Can you work these out from the model? Positions are in its coordinate system, mm. A direction names the side the tool comes from. Coordinates: 2 decimals unless noted, no trailing zeros. Order: outer loops, then holes, each group sorted by start corner. A loop starts at its lowest first (then second) coordinate and runs counter-clockwise, first axis right, second up. Notation, with made-up numbers: (73, 45.25) - (127, 45.25) arc R32 cw to (127, 83.25) - close; hole circle Ø7 at (-5, -25). An arc over 180 degrees is marked (long way). Use a Markdown table: item, result. Add a question column.
(1) On a 3-axis mill with a long thin cutter (end or side, diameter ignored), from which of +Z, -Z, +X, -X, +Y, -Y can I reach the whole of each face in a straight line? I mean faces 1 (the conical face through (24.9, 0.19, 42.68)), 2 (the flat face through (14, 16, 40.64)), 3 (the cylindrical face through (17.31, -0.34, -1.55)), 4 (the flat face through (0, -1, 1)). Say none if no direction works.
(2) We'd pull the mould along Y, two halves only. Please class faces 5 (the flat face through (25.4, 0, 43)), 6 (the conical face through (24.43, -0.24, -44.03)), 7 (the cylindrical face through (13.49, 0.21, 43.18)), 8 (the flat face through (1.524, -1, -9)): pulls with the +Y half, pulls with the -Y half, needs draft (parallel to the pull), parting line crosses it, or undercut.
(3) If I drill on L1, parallel to Z at x = 2.35, y = 0; L2, parallel to X at y = 18, z = -8; L3, parallel to Z at x = 12, y = 11, over which ranges is the centre line in solid material (lowest first)? Write a range as [from, to].
(4) I want a section at A-A (x = 7.25). State how many separate pieces and enclosed holes the cut face has, and give its area (3 significant figures).
(5) For pin 1 Ø4.5 at (x, y) = (13, 14) entering from -Z; pin 2 Ø5 at (y, z) = (-1.5, -1) entering from +X; pin 3 Ø12 at (y, z) = (-18.5, -4.5) entering from +X, each with a flat end and sliding along its axis, tell me the tip position at first contact or that it passes through.
(6) I want a section at C-C (z = -16). List the corners of the cut face in (x, y) for me.
```python
from build123d import *

# Parameters (mm, degrees)
F0_R       = 44.45
F1_DEPTH   = 25.4
F2_R       = 43.18
F3_DEPTH   = 22.86
F4_R       = 44.45
F4_R_2     = 42.545
F5_DEPTH   = 1.27
F6_W       = 25.4
F6_H       = 81.28
F7_DEPTH   = 63.5
F8_SIZE2   = 0.340285
F8_SIZE    = 1.26999
F8_2_SIZE2 = 0.340285
F8_2_SIZE  = 1.26999
F9_SIZE2   = 0.6805909488
F9_SIZE    = 2.54
F10_R      = 0.254
F11_R      = 41.91
F12_DEPTH  = 1.016
F13_R      = 4.7625
F14_DEPTH  = 9.525
F15_R      = 1.5875
F16_DEPTH  = 12.7


# Not quite as in the source:
# - a fillet or chamfer is up to 0.001 mm smaller than in the source, because OpenCascade refuses the exact size


with BuildPart() as f1:
    # F0 (on Right) → F1 (new body)
    with BuildSketch(Plane.YZ):
        Circle(F0_R)
    extrude(amount=F1_DEPTH)

    # F2 (on face) → F3 (cut)
    with BuildSketch(Plane.YZ.offset(25.4)):
        Circle(F2_R)
    extrude(amount=-F3_DEPTH, mode=Mode.SUBTRACT)

    # F4 (on face) → F5 (join)
    with BuildSketch(Plane.YZ.offset(25.4)):
        Circle(F4_R)
        Circle(F4_R_2, mode=Mode.SUBTRACT)
    extrude(amount=-F5_DEPTH)

    # F6 (on Front) → F7 (cut, symmetric)
    with BuildSketch(Plane.XZ):
        with Locations((15.24, 0)):
            Rectangle(F6_W, F6_H)
    extrude(amount=F7_DEPTH, both=True, mode=Mode.SUBTRACT)

    # F8 (size 1.27 and 0.3402954744 in the source; OpenCascade refuses exactly that, so slightly less here)
    f8_edges = [f1.edges().sort_by_distance(p)[0] for p in [
        (24.13, 0, -42.545),
    ]]
    f8_side = f1.faces().sort_by_distance((24.765, 0, -42.545))[0]
    chamfer(f8_edges, length=F8_SIZE, length2=F8_SIZE2, reference=f8_side)

    # F8#2 (size 1.27 and 0.3402954744 in the source; OpenCascade refuses exactly that, so slightly less here)
    f8_2_edges = [f1.edges().sort_by_distance(p)[0] for p in [
        (24.13, 0, 42.545),
    ]]
    f8_2_side = f1.faces().sort_by_distance((24.765, 0, 42.545))[0]
    chamfer(f8_2_edges, length=F8_2_SIZE, length2=F8_2_SIZE2, reference=f8_2_side)

    # F9
    f9_edges = [f1.edges().sort_by_distance(p)[0] for p in [
        (25.4, 0, -44.45),
        (25.4, 0, 44.45),
    ]]
    f9_side = f1.faces().sort_by_distance((1.257363, 37.256816, -24.243188))[0]
    chamfer(f9_edges, length=F9_SIZE, length2=F9_SIZE2, reference=f9_side)

    # F10
    f10_edges = [f1.edges().sort_by_distance(p)[0] for p in [
        (12.7, 18.005358, -40.64),
        (12.7, -18.005358, -40.64),
        (12.7, -18.005358, 40.64),
        (12.7, 18.005358, 40.64),
    ]]
    fillet(f10_edges, radius=F10_R)

    # F11 (on face) → F12 (cut)
    with BuildSketch(Plane.YZ.offset(2.54)):
        Circle(F11_R)
    extrude(amount=-F12_DEPTH, mode=Mode.SUBTRACT)

    # F13 (on face) → F14 (join)
    with BuildSketch(Plane.YZ.offset(1.524)):
        Circle(F13_R)
    extrude(amount=F14_DEPTH)

    # F15 (on face) → F16 (join)
    with BuildSketch(Plane.YZ.offset(11.049)):
        Circle(F15_R)
    extrude(amount=F16_DEPTH)


solid = f1.part
```
Answers follow:
| question | item | result |
|---|---|---|
| 1 | face 1 | none |
| 1 | face 2 | +X, +Y, -Y |
| 1 | face 3 | +X |
| 1 | face 4 | +Z, -Z, -X, +Y, -Y |
| 2 | face 5 | needs draft |
| 2 | face 6 | parting line crosses it |
| 2 | face 7 | undercut |
| 2 | face 8 | undercut |
| 3 | L1 | z = [-44.45, -41.91], [-4.76, 4.76], [41.91, 44.45] |
| 3 | L2 | x = [0, 1.52] |
| 3 | L3 | z = [-43.07, -41.76], [41.76, 43.07] |
| 4 | separate pieces | 3 |
| 4 | enclosed holes | 0 |
| 4 | area | 155 mm² |
| 5 | pin 1 | stops at z = -42.87 |
| 5 | pin 2 | stops at x = 23.75 |
| 5 | pin 3 | stops at x = 1.52 |
| 6 | outline | (0, -41.47) - (2.54, -41.47) - (2.54, -38.74) - (1.52, -38.74) - (1.52, 38.74) - (2.54, 38.74) - (2.54, 41.47) - (0, 41.47) - close |
